```python
from build123d import *

# Parameters (mm, degrees)
F0_W        = 61
F0_H        = 43
F1_DEPTH    = 9
F2_T1_DEPTH = 86


# Not quite as in the source:
# - a fillet or chamfer that OpenCascade refuses, or shapes differently, is made with other operations: its cross-section is extruded or revolved along the edge and cut away or added


with BuildPart() as f1:
    # F0 (on Top) → F1 (new body)
    with BuildSketch(Plane.XY):
        Rectangle(F0_W, F0_H)
    extrude(amount=F1_DEPTH)

    # F2: fillet of radius 5 on 4 edges, made by hand

    # F2_s2 → F2_t1 (cut)
    with BuildSketch(Plane.YZ.offset(-43)):
        with BuildLine():
            ThreePointArc((21.5, 4), (20.0355339059, 7.5355339059), (16.5, 9))
            Line((16.5, 9), (21.5, 9))
            Line((21.5, 9), (21.5, 4))
        make_face()
        with BuildLine():
            ThreePointArc((-21.5, 4), (-20.0355339059, 7.5355339059), (-16.5, 9))
            Line((-16.5, 9), (-21.5, 9))
            Line((-21.5, 9), (-21.5, 4))
        make_face()
        with BuildLine():
            ThreePointArc((-21.5, 5), (-20.0355339059, 1.4644660941), (-16.5, 0))
            Line((-16.5, 0), (-21.5, 0))
            Line((-21.5, 0), (-21.5, 5))
        make_face()
        with BuildLine():
            ThreePointArc((21.5, 5), (20.0355339059, 1.4644660941), (16.5, 0))
            Line((16.5, 0), (21.5, 0))
            Line((21.5, 0), (21.5, 5))
        make_face()
    extrude(amount=F2_T1_DEPTH, mode=Mode.SUBTRACT)


solid = f1.part
```
Read the model definition and answer for the solid it produces. Units are mm, in the model's axes. Coordinates: 2 decimals unless noted, no trailing zeros. Loops run counter-clockwise (first coordinate to the right, second up) from the corner with the lowest first, then second, coordinate; pieces in that order, holes last.
(1) Consider line 1 along Y through (x, z) = (-2, 3.75); line 2 along Y through (x, z) = (-9, 0.75); line 3 along Z through (x, y) = (-5.5, 18.5). Determine where each line is inside the solid, lowest interval first.
Solution:
line 1: y = -21.34 to 21.34
line 2: y = -19.13 to 19.13
line 3: z = 0.42 to 8.58
(2) The part is cut by section B-B (z = 2). Determine the outline of the cut face in (x, y), and give its area (3 significant figures).
Solution:
outline: (-30.5, -20.5) - (30.5, -20.5) - (30.5, 20.5) - (-30.5, 20.5) - close
area: 2,500 mm2
(3) The part is cut by section A-A (x = -3.5). Determine the outline of the cut face in (y, z), and give its area (3 significant figures).
Solution:
outline: (-21.47, 4.5) arc R5 ccw to (-16.5, 0) - (16.5, 0) arc R5 ccw to (21.47, 4.5) arc R5 ccw to (16.5, 9) - (-16.5, 9) arc R5 ccw to start
area: 366 mm2
(4) The part is cut by section C-C (z = 6.25). Determine the outline of the cut face in (x, y).
Solution:
outline: (-30.5, -20.97) - (30.5, -20.97) - (30.5, 20.97) - (-30.5, 20.97) - close
(5) Flat-ended cylindrical pins translate along their axes: pin 1 Ø2 at (x, z) = (-6.5, 2) entering from -Y; pin 2 Ø5 at (x, z) = (16, 1) entering from +Y; pin 3 Ø1 at (x, z) = (19, 1.5) entering from -Y. Find the tip coordinate at first contact, or state that the pin passes through.
Solution:
pin 1: stops at y = -21.08
pin 2: stops at y = 21.27
pin 3: stops at y = -20.5
